Verification items for the finished model (mm, model axes). Coordinates: 2 decimals unless noted, no trailing zeros. Order: outer loops, then holes, each group sorted by start corner. A loop starts at its lowest first (then second) coordinate and runs counter-clockwise, first axis right, second up. Notation, with made-up numbers: (-14, 3.5) - (-9, 3.5) arc R31 cw to (-9, 38.5) - close; hole circle Ø2 at (-13, 82). An arc over 180 degrees is marked (long way). Answer as CSV lines item,"result". Start each with the question number.
1. Material ranges on L1, parallel to X at y = 0.85, z = 32; L2, parallel to X at y = 0.4, z = 12; L3, parallel to X at y = 0.7, z = 29, recorded low to high. Write a range as [from, to].
2. Section check D-D (z = -35.5). Record the cut outline in (x, y).
3. Go/stop test with flat-tipped pins: pin 1 (3 mm diameter, centred on x = -28.5, z = 32, fed in from +Y); pin 2 (0.6 mm diameter, centred on x = -35.5, y = 1.5, fed in from +Z); pin 3 (2 mm diameter, centred on x = 28.5, z = 13, fed in from +Y). Record where each tip stops, or that it passes through.
4. Section check B-B (y = 1.55). Record the cut outline in (x, z), and give its area (3 significant figures).
5. Section check A-A (z = 32). Record the cut outline in (x, y), and give its area (3 significant figures).
6. Section check C-C (x = -28.5). Record the cut outline in (y, z), and give its area (3 significant figures).
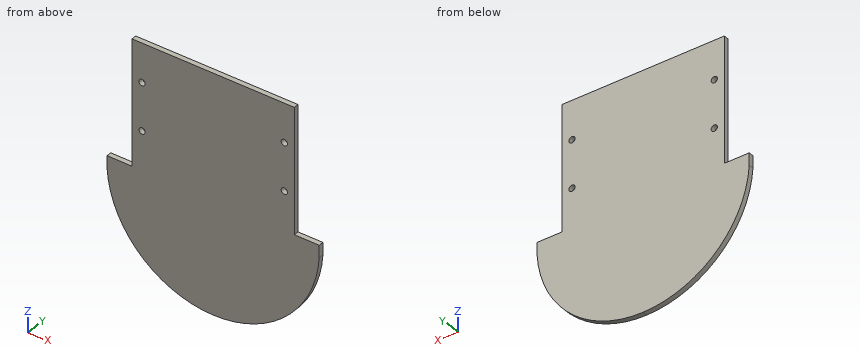
from build123d import *

# Parameters (mm, degrees)
BOSS_EXTRUDE1_DEPTH = 2
SKETCH2_R           = 1.25
CUT_EXTRUDE1_DEPTH  = 2


with BuildPart() as part:
    # Sketch1 → Boss-Extrude1 (new body)
    with BuildSketch(Plane(origin=(0, 0, 0), x_dir=(1, 0, 0), z_dir=(0, 1, 0))):
        with BuildLine():
            Line((-32.5, 2.5), (-32.5, -47.5))
            Line((-32.5, -47.5), (32.5, -47.5))
            Line((32.5, -47.5), (32.5, 2.5))
            Line((32.5, 2.5), (42.5, 2.5))
            Line((42.5, 2.5), (42.5, 7.361111111))
            ThreePointArc((42.5, 7.361111111), (29.229182401, 35.879101507), (1.65e-07, 47.5))
            ThreePointArc((1.65e-07, 47.5), (-29.229182281, 35.87910162), (-42.5, 7.361111111))
            Line((-42.5, 7.361111111), (-42.5, 2.5))
            Line((-42.5, 2.5), (-32.5, 2.5))
        make_face()
    extrude(amount=BOSS_EXTRUDE1_DEPTH)

    # Sketch2 → Cut-Extrude1 (cut)
    with BuildSketch(Plane(origin=(0, 0, 0), x_dir=(1, 0, 0), z_dir=(0, 1, 0))):
        with Locations(Location((-28.5, -13, 0), (0, 0, 270))):
            Circle(SKETCH2_R)
        with Locations(Location((-28.5, -32, 0), (0, 0, 90))):
            Circle(SKETCH2_R)
        with Locations(Location((28.5, -32, 0), (0, 0, 270))):
            Circle(SKETCH2_R)
        with Locations(Location((28.5, -13, 0), (0, 0, 90))):
            Circle(SKETCH2_R)
    extrude(amount=CUT_EXTRUDE1_DEPTH, mode=Mode.SUBTRACT)


solid = part.part
Evaluation:
1,L1,"x = [-32.5, -29.75], [-27.25, 27.25], [29.75, 32.5]"
1,L2,"x = [-32.5, -29.25], [-27.75, 27.75], [29.25, 32.5]"
1,L3,"x = [-32.5, 32.5]"
2,outline,"(-29.63, 0) - (29.63, 0) - (29.63, 2) - (-29.63, 2) - close"
3,pin 1,"stops at y = 2"
3,pin 2,"stops at z = -2.5"
3,pin 3,"passes through"
4,outline,"(-42.5, -7.36) arc R42.57 ccw to (42.5, -7.36) - (42.5, -2.5) - (32.5, -2.5) - (32.5, 47.5) - (-32.5, 47.5) - (-32.5, -2.5) - (-42.5, -2.5) - close; hole circle Ø2.5 at (-28.5, 13); hole circle Ø2.5 at (-28.5, 32); hole circle Ø2.5 at (28.5, 13); hole circle Ø2.5 at (28.5, 32)"
4,area,"6,280 mm²"
5,outline,"(-32.5, 0) - (-29.75, 0) - (-29.75, 2) - (-32.5, 2) - close; (-27.25, 0) - (27.25, 0) - (27.25, 2) - (-27.25, 2) - close; (29.75, 0) - (32.5, 0) - (32.5, 2) - (29.75, 2) - close"
5,area,"120 mm²"
6,outline,"(0, -36.55) - (2, -36.55) - (2, 11.75) - (0, 11.75) - close; (0, 14.25) - (2, 14.25) - (2, 30.75) - (0, 30.75) - close; (0, 33.25) - (2, 33.25) - (2, 47.5) - (0, 47.5) - close"
6,area,"158 mm²"
